Read the model definition and answer for the solid it produces. Units are mm, in the model's axes. A direction names the side the tool comes from. Coordinates: 2 decimals unless noted, no trailing zeros. Loops run counter-clockwise (first coordinate to the right, second up) from the corner with the lowest first, then second, coordinate; pieces in that order, holes last. Notation, with made-up numbers: (4, 38.25) - (23, 38.25) arc R37 ccw to (23, 74.25) - close; hole circle Ø6 at (33.5, 5.25). An arc over 180 degrees is marked (long way). Use one line per item in the form item = value. Start each with the question number.
1) A cutting plane is placed at C-C (x = 11.5). Give the vertices of the cut face in (y, z).
2) Each of these flat-tipped pins is pushed along its axis until it touches: P1, Ø8, axis at x = -20, z = 1, coming from the +Y side; P2, Ø4, axis at y = 16.5, z = 4.5, coming from the -X side; P3, Ø12, axis at x = 18.5, z = -9.5, coming from the -Y side; P4, Ø3, axis at x = 0, y = 0, coming from the +Z side. Where does it stop, or does it pass through?
3) Consider line 1 (Y direction, x = -6, z = 4); line 2 (X direction, y = 0, z = 8.5). Determine where each line is inside the solid, lowest interval first.
4) Which of the six approach directions +Z, -Z, +X, -X, +Y, -Y give full straight-line access (tool end or side, diameter ignored) to faces 5 (the face through (-18, -5, -5)), 6 (the face through (-25, -7, -15)), 7 (the face through (-13.967, -8.064, 0.07)), 8 (the face through (0, -3, 7.5))?
5) The mould has two halves that part along X. Classify faces 1 (the face through (-1.32, -29.97, -0.21)), 2 (the face through (-25, 7, 15)), 3 (the face through (13, -13, -5)), 4 (the face through (8.2, 14.2, 0.1)): released by +X, released by -X, zero draft, split by the parting line, or undercut.
6) A cutting plane is placed at B-B (y = -16.5). Give the vertices of the cut face in (x, z).
7) A cutting plane is placed at D-D (y = -10). Give the vertices of the cut face in (x, z), and give its area (3 significant figures).
8) A cutting plane is placed at A-A (z = -3.5). Give the vertices of the cut face in (x, y), and give its area (3 significant figures).
from build123d import *
from build123d.topology import SkipClean

# Parameters (mm, degrees)
CUT_EXTRUDE1_DEPTH = 47.904157598234306
CIRPATTERN2_COUNT  = 3
SKETCH8_R          = 2.6000000000000005
CUT_EXTRUDE2_DEPTH = 49.02343178074637


with BuildPart() as part:
    # Sketch5 → Revolve2 (revolve)
    with BuildSketch(Plane(origin=(0, 0, 0), x_dir=(0, 0, -1), z_dir=(1, 0, 0))):
        Polygon((-5.000000000000004, 7.5), (-5.000000000000003, 25), (-14.999999999999998, 24.999999999999996), (-14.999999999999998, 30), (14.999999999999998, 30), (14.999999999999998, 24.999999999999996), (5.000000000000003, 25), (5.000000000000004, 7.5), (7.5, 7.499999999999998), (7.499999999999998, -4.8e-16), (-7.499999999999998, -4.8e-16), (-7.5, 7.499999999999998), align=None)
    revolve(axis=Axis((0, 7.4e-16, -11.452014829998802), (0, -1.8e-16, 1)))

    # Sketch7 → Cut-Extrude1 (cut, through all)
    with SkipClean():  # the faces are left unmerged after this step: merging them gives an invalid solid
        with BuildSketch(Plane.XY.offset(5)):
            with BuildLine():
                Line((0, 7.499999999999999), (-2.7040460461e-06, 24.99999999999999))
                ThreePointArc((-2.7040460461e-06, 24.99999999999999), (-17.677670485688406, 17.67766857363911), (-25, -1.041e-14))
                Line((-25, -1.041e-14), (-7.500000000000001, -1.82e-15))
                ThreePointArc((-7.500000000000001, -1.82e-15), (-5.303300858899107, 5.303300858899106), (0, 7.499999999999999))
            make_face()
        cut_extrude1 = extrude(amount=-CUT_EXTRUDE1_DEPTH, mode=Mode.SUBTRACT)

    # CirPattern2: Cut-Extrude1 ×3 about axis
    cirpattern2_axis = Axis((4.4e-16, -2.5e-16, 0), (0, 0, 1))
    for i in range(1, CIRPATTERN2_COUNT):
        add(cut_extrude1.rotate(cirpattern2_axis, i * 360 / CIRPATTERN2_COUNT), mode=Mode.SUBTRACT)

    # Sketch8 → Cut-Extrude2 (cut, through all)
    with BuildSketch(Plane(origin=(0, 1.38e-15, -7.5), x_dir=(-1, 0, 0), z_dir=(0, 1.8e-16, -1))):
        with Locations(Location((0, 0, 0), (0, 0, 90))):
            Circle(SKETCH8_R)
    extrude(amount=-CUT_EXTRUDE2_DEPTH, mode=Mode.SUBTRACT)


solid = part.part
Found:
q1.outline = (-27.71, -15) - (-22.2, -15) - (-22.2, 15) - (-27.71, 15) - close; (-19.92, -5) - (-6.64, -5) - (-6.64, 5) - (-19.92, 5) - close; (19.92, -5) - (22.2, -5) - (22.2, -15) - (27.71, -15) - (27.71, 15) - (22.2, 15) - (22.2, 5) - (19.92, 5) - close
q2.P1 = 25.38
q2.P2 = -26.26
q2.P3 = -27.27
q2.P4 = through
q3.line_1 = -29.39 to -24.27, -4.5 to 4.5, 24.27 to 29.39
q3.line_2 = -30 to -25, 25 to 30
q4.face_5 = -Z
q4.face_6 = -Z, +X, -X, +Y, -Y
q4.face_7 = +Z, -Z
q4.face_8 = +Z
q5.face_1 = split by the parting line
q5.face_2 = zero draft
q5.face_3 = undercut
q5.face_4 = undercut
q6.outline = (-25.05, -15) - (-18.78, -15) - (-18.78, 15) - (-25.05, 15) - close; (9.53, -5) - (18.78, -5) - (18.78, -15) - (25.05, -15) - (25.05, 15) - (18.78, 15) - (18.78, 5) - (9.53, 5) - close
q7.outline = (-28.28, -15) - (-22.91, -15) - (-22.91, -5) - (-17.32, -5) - (-17.32, 5) - (-22.91, 5) - (-22.91, 15) - (-28.28, 15) - close; (5.77, -5) - (17.32, -5) - (17.32, 5) - (5.77, 5) - close; (22.91, -15) - (28.28, -15) - (28.28, 15) - (22.91, 15) - close
q7.area = 494 mm^2
q8.outline = circle Ø60 at (0, 0); hole (-25, 0) - (-7.5, 0) arc R7.5 cw to (0, 7.5) - (0, 25) arc R25 ccw to start; hole (-21.65, -12.5) arc R25 ccw to (12.5, -21.65) - (3.75, -6.5) arc R7.5 cw to (-6.5, -3.75) - close; hole circle Ø5.2 at (0, 0); hole (3.75, 6.5) arc R7.5 cw to (6.5, -3.75) - (21.65, -12.5) arc R25 ccw to (12.5, 21.65) - close
q8.area = 1,470 mm^2
